Read the model definition and answer for the solid it produces. Units are mm, in the model's axes. Face numbers are marked on the shaded views. A direction names the side the tool comes from. Coordinates: 2 decimals unless noted, no trailing zeros. Write each loop counter-clockwise with the first axis right and the second up, starting at its lowest first coordinate (ties: lowest second). Pieces come first, ordered by that corner, then holes.
1) Find the intervals of material crossed by line 1 (X direction, y = -7.5, z = 7.5); line 2 (Z direction, x = 68.5, y = 0); line 3 (X direction, y = 0.75, z = 6.25), in increasing order.
2) The part is cut by section C-C (z = -6.5). Determine the outline of the cut face in (x, y) (3 decimals).
3) The part is cut by section B-B (y = -7). Determine the outline of the cut face in (x, z).
4) The part is cut by section A-A (x = -5). Determine the outline of the cut face in (y, z) (3 decimals).
5) Which of the six approach directions +Z, -Z, +X, -X, +Y, -Y give full straight-line access (tool end or side, diameter ignored) to the marked faces 1, 2 and 3?
6) The part is cut by section D-D (x = 25.5). Determine the outline of the cut face in (y, z), then the cut area to 3 significant figures.
7) Determine the mould class of the marked faces 4, 5, 6 and 7 for opening direction X: +X half, -X half, draft (parallel to the pull), parting line (faces both ways), or undercut.
8) Each of these flat-tipped pins is pushed along its axis until it touches: pin 1 Ø1 at (x, z) = (55.5, 6) entering from -Y; pin 2 Ø1 at (x, z) = (20.5, 11.5) entering from -Y; pin 3 Ø3 at (y, z) = (-1.5, 13.5) entering from -X; pin 4 Ø2.5 at (x, y) = (2.57, 0) entering from +Z. Where does it stop, or does it pass through?
from build123d import *

# Parameters (mm, degrees)
F0_W      = 5.842
F0_H      = 12.7
F0_R      = 3.175
F2_DEPTH  = 3.175
F3_DEPTH  = 6.35
F4_R      = 1.524
F5_DEPTH  = 7.62
F6_DEPTH  = 1.27
F8_R      = 1.524
F9_DEPTH  = 10.414
F7_R      = 1.524
F10_DEPTH = 17.78


with BuildPart() as f1:
    # F0 (on Front) → F1 (revolve)
    with BuildSketch(Plane.XZ):
        Polygon((5.842, 12.7), (5.842, 0), (66.294, 0), (66.294, 12.7), (56.134, 12.7), (56.134, 10.16), (10.16, 10.16), (10.16, 12.7), align=None)
        with Locations((2.921, 6.35)):
            Rectangle(F0_W, F0_H)
    revolve(axis=Axis((33.147, 0, 0), (-1, 0, 0)))

    # F0 (on Front) → F2 (join)
    with BuildSketch(Plane.XZ):
        with BuildLine():
            Line((-0.9398, 0), (0, 0))
            Line((0, 0), (0, 12.7))
            Line((0, 12.7), (5.842, 12.7))
            Line((5.842, 12.7), (5.842, 15.24))
            Line((5.842, 15.24), (-0.508, 15.24))
            Line((-0.508, 15.24), (-10.8806298187, 3.8475430269))
            ThreePointArc((-10.8806298187, 3.8475430269), (-4.5919612295, 5.3297205562), (-0.9398, 0))
        make_face()
        with BuildLine():
            ThreePointArc((-8.1826630726, -5.5069827884), (-3.1957909266, -4.5493385486), (-0.9398, 0))
            ThreePointArc((-0.9398, 0), (-4.5919612295, 5.3297205562), (-10.8806298187, 3.8475430269))
            ThreePointArc((-10.8806298187, 3.8475430269), (-12.1459778134, -1.5837270034), (-8.1826630726, -5.5069827884))
        make_face()
        with Locations((-6.6548, 0)):
            Circle(F0_R, mode=Mode.SUBTRACT)
        with BuildLine():
            Line((5.842, 0), (0, 0))
            Line((0, 0), (-0.9398, 0))
            ThreePointArc((-0.9398, 0), (-3.1957909266, -4.5493385486), (-8.1826630726, -5.5069827884))
            Line((-8.1826630726, -5.5069827884), (5.842, -9.398))
            Line((5.842, -9.398), (5.842, 0))
        make_face()
        with Locations((2.921, 6.35)):
            Rectangle(F0_W, F0_H)
    extrude(amount=F2_DEPTH)

    # F3 (add): a face of the model
    f3_faces = [f1.faces().sort_by_distance(p)[0] for p in [
        (-3.7379712186, -3.175, 3.6396098822),
    ]]
    extrude(f3_faces, amount=-F3_DEPTH)

    # F4 (on face) → F5 (join)
    with BuildSketch(Plane.YZ.offset(66.294)):
        with BuildLine():
            ThreePointArc((-5.0794025007, 0.0779117191), (-0.0389570051, -5.079850623), (5.08, 0))
            ThreePointArc((5.08, 0), (5.0799978531, 0.0046703639), (5.0799914125, 0.0093407238))
            ThreePointArc((5.0799914125, 0.0093407238), (0.0342867621, 5.0798842918), (-5.0794025007, 0.0779117191))
        make_face()
        Circle(F4_R, mode=Mode.SUBTRACT)
        with BuildLine():
            ThreePointArc((-5.0794025007, 0.0779117191), (0.0342867621, 5.0798842918), (5.0799914125, 0.0093407238))
            Line((5.0799914125, 0.0093407238), (5.0799914125, 11.6397460131))
            ThreePointArc((5.0799914125, 11.6397460131), (0.0003212741, 12.6999999959), (-5.0794025007, 11.640003017))
            Line((-5.0794025007, 11.640003017), (-5.0794025007, 0.0779117191))
        make_face()
        with BuildLine():
            ThreePointArc((-5.0794025007, 11.640003017), (0.0003212741, 12.6999999959), (5.0799914125, 11.6397460131))
            Line((5.0799914125, 11.6397460131), (5.0799914125, 15.2493407238))
            Line((5.0799914125, 15.2493407238), (-5.0794025007, 15.3179117191))
            Line((-5.0794025007, 15.3179117191), (-5.0794025007, 11.640003017))
        make_face()
    extrude(amount=F5_DEPTH)

    # F6 (add): a face of the model
    f6_faces = [f1.faces().sort_by_distance(p)[0] for p in [
        (66.294, -0.0194413751, 13.8014276959),
    ]]
    extrude(f6_faces, amount=F6_DEPTH)

    # F8 (on face) → F9 (cut)
    with BuildSketch(Plane(origin=(0, 0.1031523992, 15.2829319801), x_dir=(1, 0, 0), z_dir=(0, 0.0067493626, 0.9999772228))):
        with Locations((69.469, -0.1028602862)):
            Circle(F8_R)
    extrude(amount=-F9_DEPTH, mode=Mode.SUBTRACT)

    # F7 (on face) → F10 (cut)
    with BuildSketch(Plane.XY.offset(15.24)):
        with Locations((2.5670649484, 0)):
            Circle(F7_R)
    extrude(amount=-F10_DEPTH, mode=Mode.SUBTRACT)


solid = f1.part
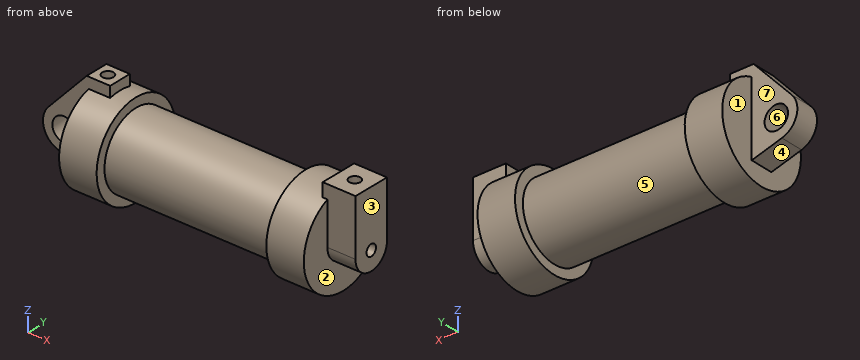
Reported:
1. line 1: x = 0 to 10.16, 56.13 to 66.29
1. line 2: z = -5.08 to -1.52, 1.52 to 4.87
1. line 3: x = -8.69 to 1.24, 3.89 to 68.18, 70.76 to 73.91
2. outline: (-4.603, -3.175) - (0, -3.175) - (0, -10.911) - (10.16, -10.911) - (10.16, -7.809) - (56.134, -7.809) - (56.134, -10.911) - (66.294, -10.911) - (66.294, 10.911) - (56.134, 10.911) - (56.134, 7.809) - (10.16, 7.809) - (10.16, 10.911) - (0, 10.911) - (0, 3.175) - (-4.603, 3.175) - close
3. outline: (0, -10.6) - (10.16, -10.6) - (10.16, -7.36) - (56.13, -7.36) - (56.13, -10.6) - (66.29, -10.6) - (66.29, 10.6) - (56.13, 10.6) - (56.13, 7.36) - (10.16, 7.36) - (10.16, 10.6) - (0, 10.6) - close
4. outline: (-3.175, -6.39) - (3.175, -6.39) - (3.175, -2.71) - (-3.175, -2.71) - close; (-3.175, 2.71) - (3.175, 2.71) - (3.175, 10.306) - (-3.175, 10.306) - close
5. face 1: -Z, -X
5. face 2: -Z, +X
5. face 3: +Z, -Z, +X, +Y, -Y
6. outline: circle Ø20.32 at (0, 0)
6. area: 324 mm2
7. face 4: -X half
7. face 5: undercut
7. face 6: undercut
7. face 7: draft
8. pin 1: stops at y = -8.54
8. pin 2: passes through
8. pin 3: stops at x = -3.46
8. pin 4: stops at z = -2.54
